from build123d import *

# Parameters (mm, degrees)
BOSS_EXTRUDE1_DEPTH   = 5.715
CUT_EXTRUDE1_DEPTH    = 6.715
F_6_CLEARANCE_HOLE1_D = 3.7973


with BuildPart() as part:
    # Model → Boss-Extrude1 (new body)
    with BuildSketch(Plane.XY):
        Polygon((1382.75, 22.8575), (1396.32, 22.8575), (1396.32, 28.5722), (1407.75, 28.5722), (1407.75, 22.8575), (1419.18, 22.8575), (1419.18, 28.5722), (1430.61, 28.5722), (1430.61, 22.8575), (1442.04, 22.8575), (1442.04, 28.5722), (1453.47, 28.5722), (1453.47, 22.8575), (1464.9, 22.8575), (1464.9, 28.5722), (1476.33, 28.5722), (1476.33, 22.8575), (1487.76, 22.8575), (1487.76, 28.5722), (1499.19, 28.5722), (1499.19, 22.8575), (1510.62, 22.8575), (1510.62, 28.5722), (1522.05, 28.5722), (1522.05, 22.8575), (1535.61, 22.8575), (1535.61, 28.5722), (1535.61, 51.4325), (1535.61, 51.8072), (1535.51, 52.9276), (1535.22, 54.3913), (1534.74, 55.8038), (1534.27, 56.8247), (1534.08, 57.1472), (1533.99, 57.3098), (1533.68, 57.7854), (1533.25, 58.3928), (1532.77, 58.9703), (1532.27, 59.5147), (1531.72, 60.0244), (1531.14, 60.4986), (1530.53, 60.9353), (1530.06, 61.2387), (1529.9, 61.3311), (1529.74, 61.4246), (1529.26, 61.728), (1528.65, 62.1647), (1528.07, 62.6389), (1527.53, 63.1486), (1527.02, 63.693), (1526.55, 64.2705), (1526.11, 64.878), (1525.81, 65.3535), (1525.71, 65.5147), (1525.53, 65.8386), (1525.05, 66.8595), (1524.57, 68.272), (1524.28, 69.7357), (1524.18, 70.8561), (1524.18, 71.2294), (1524.18, 245.915), (1524.18, 246.29), (1524.28, 247.41), (1524.57, 248.874), (1525.05, 250.286), (1525.53, 251.307), (1525.71, 251.63), (1525.81, 251.792), (1526.11, 252.268), (1526.55, 252.876), (1527.02, 253.453), (1527.53, 253.997), (1528.07, 254.507), (1528.65, 254.981), (1529.26, 255.418), (1529.74, 255.72), (1529.9, 255.814), (1530.06, 255.907), (1530.53, 256.211), (1531.14, 256.647), (1531.72, 257.121), (1532.27, 257.631), (1532.77, 258.175), (1533.25, 258.753), (1533.68, 259.36), (1533.99, 259.836), (1534.08, 259.997), (1534.27, 260.321), (1534.74, 261.342), (1535.22, 262.755), (1535.51, 264.218), (1535.61, 265.339), (1535.61, 265.712), (1535.61, 288.572), (1535.61, 294.287), (1522.05, 294.287), (1522.05, 288.572), (1510.62, 288.572), (1510.62, 294.287), (1499.19, 294.287), (1499.19, 288.572), (1487.76, 288.572), (1487.76, 294.287), (1476.33, 294.287), (1476.33, 288.572), (1464.9, 288.572), (1464.9, 294.287), (1453.47, 294.287), (1453.47, 288.572), (1442.04, 288.572), (1442.04, 294.287), (1430.61, 294.287), (1430.61, 288.572), (1419.18, 288.572), (1419.18, 294.287), (1407.75, 294.287), (1407.75, 288.572), (1396.32, 288.572), (1396.32, 294.287), (1382.75, 294.287), (1382.75, 288.572), (1382.75, 28.5722), align=None)
        Polygon((1518.47, 44.2722), (1518.47, 38.5576), (1512.75, 38.5576), (1512.75, 49.9868), (1518.47, 49.9868), align=None, mode=Mode.SUBTRACT)
        Polygon((1518.47, 67.1326), (1518.47, 61.4179), (1512.75, 61.4179), (1512.75, 72.8472), (1518.47, 72.8472), align=None, mode=Mode.SUBTRACT)
        Polygon((1518.47, 89.9929), (1518.47, 84.2779), (1512.75, 84.2779), (1512.75, 95.7076), (1518.47, 95.7076), align=None, mode=Mode.SUBTRACT)
        Polygon((1518.47, 112.853), (1518.47, 107.137), (1512.75, 107.137), (1512.75, 118.568), (1518.47, 118.568), align=None, mode=Mode.SUBTRACT)
        Polygon((1518.47, 135.712), (1518.47, 129.997), (1512.75, 129.997), (1512.75, 141.428), (1518.47, 141.428), align=None, mode=Mode.SUBTRACT)
        Polygon((1518.47, 158.572), (1518.47, 152.858), (1512.75, 152.858), (1512.75, 164.287), (1518.47, 164.287), align=None, mode=Mode.SUBTRACT)
        Polygon((1518.47, 181.433), (1518.47, 175.718), (1512.75, 175.718), (1512.75, 187.147), (1518.47, 187.147), align=None, mode=Mode.SUBTRACT)
        Polygon((1518.47, 204.293), (1518.47, 198.578), (1512.75, 198.578), (1512.75, 210.008), (1518.47, 210.008), align=None, mode=Mode.SUBTRACT)
        Polygon((1518.47, 227.153), (1518.47, 221.437), (1512.75, 221.437), (1512.75, 232.868), (1518.47, 232.868), align=None, mode=Mode.SUBTRACT)
        Polygon((1518.47, 250.012), (1518.47, 244.297), (1512.75, 244.297), (1512.75, 255.728), (1518.47, 255.728), align=None, mode=Mode.SUBTRACT)
        Polygon((1518.47, 272.872), (1518.47, 267.158), (1512.75, 267.158), (1512.75, 278.587), (1518.47, 278.587), align=None, mode=Mode.SUBTRACT)
    extrude(amount=BOSS_EXTRUDE1_DEPTH)

    # Sketch1 → Cut-Extrude1 (cut, through all)
    with BuildSketch(Plane(origin=(0, 0, 0), x_dir=(-1, 0, 0), z_dir=(0, 0, -1))):
        with BuildLine():
            Line((-1468.0398, 277.5723), (-1507.5398, 277.5723))
            Line((-1507.5398, 277.5723), (-1507.5398, 189.5723))
            Line((-1507.5398, 189.5723), (-1468.0398, 189.5723))
            Line((-1468.0398, 189.5723), (-1468.0398, 193.624933404))
            ThreePointArc((-1468.0398, 193.624933404), (-1466.960094146, 194.312961338), (-1466.5398, 195.5223))
            Line((-1466.5398, 195.5223), (-1466.5398, 234.6223))
            ThreePointArc((-1466.5398, 234.6223), (-1466.960094146, 235.831638662), (-1468.0398, 236.519666596))
            Line((-1468.0398, 236.519666596), (-1468.0398, 277.5723))
        make_face()
    extrude(amount=-CUT_EXTRUDE1_DEPTH, mode=Mode.SUBTRACT)

    # #6 Clearance Hole1 (through all)
    with Locations(Plane(origin=(0, 0, 0), x_dir=(-1, 0, 0), z_dir=(0, 0, -1))):
        with Locations((-1400.25, 246.0721), (-1400.25, 191.0721), (-1400.25, 126.0721), (-1400.25, 71.0721), (-1457.2548, 274.072), (-1457.2548, 229.072), (-1457.2548, 184.072), (-1495.2548, 147.02225), (-1495.2548, 102.02225), (-1495.2548, 57.02225)):
            Hole(F_6_CLEARANCE_HOLE1_D / 2)


solid = part.part
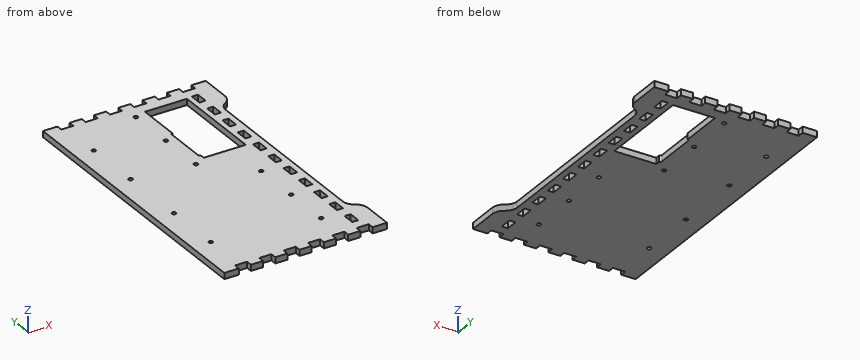
Read the model definition and answer for the solid it produces. Units are mm, in the model's axes. Give positions to 0.01 mm unless a question says otherwise; leave off trailing zeros. Loops run counter-clockwise (first coordinate to the right, second up) from the corner with the lowest first, then second, coordinate; pieces in that order, holes last. Notation, with made-up numbers: (86, -14.75) - (119, -14.75) arc R21 ccw to (119, 15.25) - close; hole circle Ø1 at (0, 30). An arc over 180 degrees is marked (long way). Answer as CSV lines item,"result". Start each with the question number.
1) Find section A-A (y = 161). Write down the section's boundary in (x, z) (3 decimals), then the cut area to 3 significant figures.
2) Straight lines are drawn through the part: L1, parallel to Y at x = 1400.25, z = 3.75; L2, parallel to X at y = 45.5, z = 0.65; L3, parallel to X at y = 205.5, z = 4.55. For each, find the intervals that lie inside material, in ascending order. Write a range as from..to.
3) Find section B-B (z = 1.95). State how many separate pieces and enclosed holes the cut face has, then the cut area to 3 significant figures.
4) Each of these flat-tipped pins is pushed along its axis until it touches: pin 1 Ø3 at (x, z) = (1495, 3.5) entering from -Y; pin 2 Ø3 at (y, z) = (161.5, 1.5) entering from +X; pin 3 Ø1.7 at (x, z) = (1473, 3.5) entering from +Y. Where does it stop, or does it pass through?
Findings below:
1,outline,"(1382.75, 0) - (1512.75, 0) - (1512.75, 5.715) - (1382.75, 5.715) - close; (1518.47, 0) - (1524.18, 0) - (1524.18, 5.715) - (1518.47, 5.715) - close"
1,area,"776 mm^2"
2,L1,"28.57..69.17, 72.97..124.17, 127.97..189.17, 192.97..244.17, 247.97..288.57"
2,L2,"1382.75..1512.75, 1518.47..1535.61"
2,L3,"1382.75..1466.54, 1507.54..1512.75, 1518.47..1524.18"
3,separate pieces,"1"
3,enclosed holes,"22"
3,area,"34,100 mm^2"
4,pin 1,"y = 28.57"
4,pin 2,"x = 1524.18"
4,pin 3,"y = 288.57"
